Here's how the part is built. I have some questions about the finished solid (model axes, mm). A direction names the side the tool comes from. Round coordinates to 2 decimals unless told otherwise and drop trailing zeros. Write each loop counter-clockwise with the first axis right and the second up, starting at its lowest first coordinate (ties: lowest second). Pieces come first, ordered by that corner, then holes. Notation, with made-up numbers: (78, -25.5) -> (119, -25.5) arc R20 cw to (119, -14.5) -> close; hole circle Ø2 at (6, 62). An arc over 180 degrees is marked (long way). Answer in a Markdown table with one row per item.
from build123d import *

# Parameters (mm, degrees)
SALIENTE_EXTRUIR1_DEPTH = 20
CROQUIS2_W              = 5.2
CROQUIS2_H              = 5.2
SALIENTE_EXTRUIR2_DEPTH = 9
CROQUIS3_W              = 5.2
CROQUIS3_H              = 16
SALIENTE_EXTRUIR4_DEPTH = 2
REDONDEO4_R             = 2.5


with BuildPart() as part:
    # Croquis1 → Saliente-Extruir1 (new body)
    with BuildSketch(Plane.XY):
        Polygon((-5.5, 0), (5.5, 0), (5.5, -2.5), (2.6, -2.5), (2.6, -5), (-2.6, -5), (-2.6, -2.5), (-5.5, -2.5), align=None)
    extrude(amount=SALIENTE_EXTRUIR1_DEPTH)

    # Croquis2 → Saliente-Extruir2 (add)
    with BuildSketch(Plane.XZ.offset(5)):
        with Locations((0, 9.535930778)):
            Rectangle(CROQUIS2_W, CROQUIS2_H)
    extrude(amount=SALIENTE_EXTRUIR2_DEPTH)

    # Croquis3 → Saliente-Extruir4 (add)
    with BuildSketch(Plane.XZ.offset(14)):
        with Locations((0, 9.535930778)):
            Rectangle(CROQUIS3_W, CROQUIS3_H)
    extrude(amount=SALIENTE_EXTRUIR4_DEPTH)

    # Redondeo4
    redondeo4_edges = [part.edges().sort_by_distance(p)[0] for p in [
        (-2.6, -9.5, 12.135930778),
        (-2.6, -9.5, 6.935930778),
        (2.6, -9.5, 6.935930778),
        (2.6, -9.5, 12.135930778),
    ]]
    fillet(redondeo4_edges, radius=REDONDEO4_R)


solid = part.part
1) We'd pull the mould along Y, two halves only. Please class faces 5 (the face through (0, -14, 5)), 6 (the face through (4, -2.5, 10)), 7 (the face through (5.5, -1, 10)): +Y half, -Y half, draft (parallel to the pull), parting line (faces both ways), or undercut.
Response:
| item | result |
|---|---|
| face 5 | undercut |
| face 6 | -Y half |
| face 7 | draft |
2) I need wall thicknesses on line 1 (Y direction, x = 1.75, z = 12.25); line 2 (X direction, y = -14.25, z = 3.25); line 3 (Y direction, x = -0.25, z = 19.25). Which ranges of each line are inside material? Lowest first, please. Write a range as [from, to].
Response:
| item | result |
|---|---|
| line 1 | y = [-16, -14], [-5, 0] |
| line 2 | x = [-2.6, 2.6] |
| line 3 | y = [-5, 0] |
3) For pin 1 (1.5 mm diameter, centred on x = 0, y = -8.5, fed in from +Z); pin 2 (5 mm diameter, centred on x = 3, y = -9, fed in from -Z); pin 3 (1.6 mm diameter, centred on x = 0, y = -15, fed in from -Z), each with a flat end and sliding along its axis, tell me the tip position at first contact or that it passes through.
Response:
| item | result |
|---|---|
| pin 1 | stops at z = 12.14 |
| pin 2 | stops at z = 6.97 |
| pin 3 | stops at z = 1.54 |
4) I want a section at C-C, the plane x = -2.25. List the corners of the cut face in (y, z) for me.
Response:
| item | result |
|---|---|
| outline | (-16, 1.54) -> (-14, 1.54) -> (-14, 8.16) -> (-5, 8.16) -> (-5, 0) -> (0, 0) -> (0, 20) -> (-5, 20) -> (-5, 10.91) -> (-14, 10.91) -> (-14, 17.54) -> (-16, 17.54) -> close |
5) I want a section at A-A, the plane z = 5.25. List the corners of the cut face in (x, y) for me.
Response:
| item | result |
|---|---|
| outline | (-5.5, -2.5) -> (-2.6, -2.5) -> (-2.6, -5) -> (2.6, -5) -> (2.6, -2.5) -> (5.5, -2.5) -> (5.5, 0) -> (-5.5, 0) -> close; (-2.6, -16) -> (2.6, -16) -> (2.6, -14) -> (-2.6, -14) -> close |
6) I want a section at D-D, the plane z = 10.25. List the corners of the cut face in (x, y) for me.
Response:
| item | result |
|---|---|
| outline | (-5.5, -2.5) -> (-2.6, -2.5) -> (-2.6, -5) -> (-2.52, -5) -> (-2.52, -14) -> (-2.6, -14) -> (-2.6, -16) -> (2.6, -16) -> (2.6, -14) -> (2.52, -14) -> (2.52, -5) -> (2.6, -5) -> (2.6, -2.5) -> (5.5, -2.5) -> (5.5, 0) -> (-5.5, 0) -> close |
7) I want a section at B-B, the plane y = -8.75. List the corners of the cut face in (x, z) for me, and give its area (3 significant figures).
Response:
| item | result |
|---|---|
| outline | (-2.6, 9.44) arc R2.5 ccw to (-0.1, 6.94) -> (0.1, 6.94) arc R2.5 ccw to (2.6, 9.44) -> (2.6, 9.64) arc R2.5 ccw to (0.1, 12.14) -> (-0.1, 12.14) arc R2.5 ccw to (-2.6, 9.64) -> close |
| area | 21.7 mm^2 |
8) Which directions (+Z, -Z, +X, -X, +Y, -Y) give clear straight access to the entire face, cutting with the end or side of a thin tool? Please do faces 1 (the face through (-1.9, -9.6, 7.7)), 2 (the face through (1.89, -9.56, 11.38)), 3 (the face through (0, -15, 17.536)), 4 (the face through (2.6, -4.7, 9.2)).
Response:
| item | result |
|---|---|
| face 1 | -Z, -X |
| face 2 | +Z, +X |
| face 3 | +Z, +X, -X, -Y |
| face 4 | +Z, -Z, +X, -Y |
